Part model, mm, in its own coordinate system. A direction names the side the tool comes from. Give positions to 0.01 mm unless a question says otherwise; leave off trailing zeros. Order: outer loops, then holes, each group sorted by start corner. A loop starts at its lowest first (then second) coordinate and runs counter-clockwise, first axis right, second up.
1. Slice it at C-C on x = 11.5. List the corners of the cut face in (y, z), and give its area (3 significant figures).
2. Which spindle directions (+Z, -Z, +X, -X, +Y, -Y) get a long thin tool onto all of the face, cutting with end or side? Do faces 1 (the flat face through (11, 12, 24)), 2 (the cylindrical face through (-13.5, -13.53, 16.76)). Say none if no direction does.
3. Drop flat-ended pins along their axis: pin 1 Ø2 at (x, y) = (-12, -11.5) entering from +Z; pin 2 Ø1.2 at (x, y) = (11, 11.5) entering from +Z; pin 3 Ø1.5 at (x, y) = (-0.5, -0.5) entering from +Z. Give the stop position or say it passes through.
4. Mould opens along X. For faces 3 (the flat face through (0, 0, 26)), 4 (the flat face through (14.1, 0, 17)), 5 (the flat face through (-11, -12, 24)), 6 (the flat face through (0, -14.1, 17)) say: +X half, -X half, draft (parallel to the pull), parting line (faces both ways), or undercut.
5. Slice it at A-A on z = 28. List the corners of the cut face in (x, y), and give its area (3 significant figures).
6. Slice it at B-B on y = 0. List the corners of the cut face in (x, z).
7. Slice it at D-D on y = -7. List the corners of the cut face in (x, z), and give its area (3 significant figures).
8. Probe line 1 (X direction, y = -11.5, z = 30.5); line 2 (Z direction, x = 8.25, y = 7.75). List the from-to ranges inside material, lowest first.
from build123d import *

# Parameters (mm, degrees)
BOSS_EXTRUDE1_DEPTH = 34
SKETCH2_R           = 11
BOSS_EXTRUDE2_DEPTH = 2
SKETCH3_R           = 2.5
CUT_EXTRUDE1_DEPTH  = 10
SKETCH4_R           = 1.25
CUT_EXTRUDE2_DEPTH  = 10


with BuildPart() as part:
    # Sketch1 → Boss-Extrude1 (new body)
    with BuildSketch(Plane.XY):
        with BuildLine():
            Line((-12.1, 14.1), (12.1, 14.1))
            ThreePointArc((12.1, 14.1), (13.514213562, 13.514213562), (14.1, 12.1))
            Line((14.1, 12.1), (14.1, -12.1))
            ThreePointArc((14.1, -12.1), (13.514213562, -13.514213562), (12.1, -14.1))
            Line((12.1, -14.1), (-12.1, -14.1))
            ThreePointArc((-12.1, -14.1), (-13.514213562, -13.514213562), (-14.1, -12.1))
            Line((-14.1, -12.1), (-14.1, 12.1))
            ThreePointArc((-14.1, 12.1), (-13.514213562, 13.514213562), (-12.1, 14.1))
        make_face()
    extrude(amount=BOSS_EXTRUDE1_DEPTH)

    # Sketch2 → Boss-Extrude2 (add)
    with BuildSketch(Plane.XY.offset(34)):
        Circle(SKETCH2_R)
    extrude(amount=BOSS_EXTRUDE2_DEPTH)

    # Sketch3 → Cut-Extrude1 (cut)
    with BuildSketch(Plane.XY.offset(36)):
        Circle(SKETCH3_R)
    extrude(amount=-CUT_EXTRUDE1_DEPTH, mode=Mode.SUBTRACT)

    # Sketch4 → Cut-Extrude2 (cut)
    with BuildSketch(Plane.XY.offset(34)):
        with Locations((-11.5, 11.5)):
            Circle(SKETCH4_R)
        with Locations((11.5, 11.5)):
            Circle(SKETCH4_R)
        with Locations(Location((11.5, -11.5, 0), (0, 0, 180))):
            Circle(SKETCH4_R)
        with Locations(Location((-11.5, -11.5, 0), (0, 0, 180))):
            Circle(SKETCH4_R)
    extrude(amount=-CUT_EXTRUDE2_DEPTH, mode=Mode.SUBTRACT)


solid = part.part
Data:
1. outline: (-14.1, 0) - (14.1, 0) - (14.1, 34) - (12.75, 34) - (12.75, 24) - (10.25, 24) - (10.25, 34) - (-10.25, 34) - (-10.25, 24) - (-12.75, 24) - (-12.75, 34) - (-14.1, 34) - close
1. area: 909 mm2
2. face 1: +Z
2. face 2: +Z, -Z, -X, -Y
3. pin 1: stops at z = 34
3. pin 2: stops at z = 24
3. pin 3: stops at z = 26
4. face 3: undercut
4. face 4: +X half
4. face 5: undercut
4. face 6: draft
5. outline: (-14.1, -12.1) arc R2 ccw to (-12.1, -14.1) - (12.1, -14.1) arc R2 ccw to (14.1, -12.1) - (14.1, 12.1) arc R2 ccw to (12.1, 14.1) - (-12.1, 14.1) arc R2 ccw to (-14.1, 12.1) - close; hole circle Ø2.5 at (-11.5, -11.5); hole circle Ø2.5 at (-11.5, 11.5); hole circle Ø5 at (0, 0); hole circle Ø2.5 at (11.5, -11.5); hole circle Ø2.5 at (11.5, 11.5)
5. area: 753 mm2
6. outline: (-14.1, 0) - (14.1, 0) - (14.1, 34) - (11, 34) - (11, 36) - (2.5, 36) - (2.5, 26) - (-2.5, 26) - (-2.5, 36) - (-11, 36) - (-11, 34) - (-14.1, 34) - close
7. outline: (-14.1, 0) - (14.1, 0) - (14.1, 34) - (8.49, 34) - (8.49, 36) - (-8.49, 36) - (-8.49, 34) - (-14.1, 34) - close
7. area: 993 mm2
8. line 1: x = -14.1 to -12.75, -10.25 to 10.25, 12.75 to 14.1
8. line 2: z = 0 to 34
